```python
from build123d import *

# Parameters (mm, degrees)
SKETCH1_W           = 26
SKETCH1_H           = 18
BOSS_EXTRUDE1_DEPTH = 4
SKETCH2_W           = 3
SKETCH2_H           = 18
BOSS_EXTRUDE2_DEPTH = 35
SKETCH3_R           = 2.75
CUT_EXTRUDE1_DEPTH  = 45.519658579
FILLET1_R           = 3
FILLET2_R           = 5
SKETCH5_R           = 7
BOSS_EXTRUDE3_DEPTH = 2
CUT_EXTRUDE3_REACH  = 44.083
SKETCH7_R           = 2.25
CUT_EXTRUDE4_DEPTH  = 4
CHAMFER1_SIZE       = 2


with BuildPart() as part:
    # Sketch1 → Boss-Extrude1 (new body)
    with BuildSketch(Plane(origin=(0, 0, 0), x_dir=(0, 0, -1), z_dir=(1, 0, 0))):
        Rectangle(SKETCH1_W, SKETCH1_H)
    extrude(amount=BOSS_EXTRUDE1_DEPTH)

    # Sketch2 → Boss-Extrude2 (add)
    with BuildSketch(Plane.ZY):
        with Locations((-11.5, 0)):
            Rectangle(SKETCH2_W, SKETCH2_H)
        with Locations((11.5, 0)):
            Rectangle(SKETCH2_W, SKETCH2_H)
    extrude(amount=BOSS_EXTRUDE2_DEPTH)

    # Sketch3 → Cut-Extrude1 (cut, through all)
    with BuildSketch(Plane.XY.offset(13)):
        with Locations((-29.5, 0)):
            Circle(SKETCH3_R)
    extrude(amount=-CUT_EXTRUDE1_DEPTH, mode=Mode.SUBTRACT)

    # Fillet1
    fillet1_edges = [part.edges().sort_by_distance(p)[0] for p in [
        (4, 0, 13),
        (0, 0, -10),
        (0, 0, 10),
        (4, 0, -13),
    ]]
    fillet(fillet1_edges, radius=FILLET1_R)

    # Fillet2
    fillet2_edges = [part.edges().sort_by_distance(p)[0] for p in [
        (-35, -9, -11.5),
        (-35, 9, -11.5),
        (-35, 9, 11.5),
        (-35, -9, 11.5),
    ]]
    fillet(fillet2_edges, radius=FILLET2_R)

    # Sketch5 → Boss-Extrude3 (add)
    with BuildSketch(Plane.ZY):
        Circle(SKETCH5_R)
    extrude(amount=BOSS_EXTRUDE3_DEPTH)

    # Sketch7 → Cut-Extrude3 (cut, up to next)
    with BuildSketch(Plane(origin=(4, 0, 0), x_dir=(0, 0, -1), z_dir=(1, 0, 0)), mode=Mode.PRIVATE) as cut_extrude3_sk1:
        Circle(SKETCH7_R)
    cut_extrude3_tool1 = extrude(cut_extrude3_sk1.sketch, amount=-CUT_EXTRUDE3_REACH, mode=Mode.PRIVATE) & part.part
    add(cut_extrude3_tool1.solids().sort_by_distance((4, 0, 0))[0], mode=Mode.SUBTRACT)

    # Sketch8 → Cut-Extrude4 (cut)
    with BuildSketch(Plane.ZY.offset(2)):
        Polygon((0, 4.330127019), (-3.75, 2.165063509), (-3.75, -2.165063509), (0, -4.330127019), (3.75, -2.165063509), (3.75, 2.165063509), align=None)
    extrude(amount=-CUT_EXTRUDE4_DEPTH, mode=Mode.SUBTRACT)

    # Chamfer1
    # the kernel refuses this chamfer: 2 mm, written as the material it adds along each edge
    with BuildSketch(Plane(origin=(0, 0, 0), x_dir=(0, 0, 1), z_dir=(0, -1, 0))) as chamfer1_piece_1_section:
        Polygon((7 + CHAMFER1_SIZE, 0), (7, CHAMFER1_SIZE), (7, 0), align=None)
    chamfer1_piece_1 = revolve(axis=Axis((0, 0, 0), (-1, 0, 0)), revolution_arc=180.000000041, mode=Mode.PRIVATE)
    chamfer1_piece_1 = split(chamfer1_piece_1, bisect_by=Plane(origin=(-0.945175713, 9, -3e-09), z_dir=(0, -1, 0)), keep=Keep.TOP, mode=Mode.PRIVATE)
    chamfer1_piece_1 = split(chamfer1_piece_1, bisect_by=Plane(origin=(-2, 8.001744255, -3e-09), z_dir=(1, 0, 0)), keep=Keep.TOP, mode=Mode.PRIVATE)
    add(chamfer1_piece_1)
    with BuildSketch(Plane(origin=(0, 0, 0), x_dir=(0, -7.23525117256177e-10, -1.0), z_dir=(0, 1.0, -7.23525117256177e-10))) as chamfer1_piece_2_section:
        Polygon((7 + CHAMFER1_SIZE, 0), (7, CHAMFER1_SIZE), (7, 0), align=None)
    chamfer1_piece_2 = revolve(axis=Axis((0, 0, 0), (-1, 0, 0)), revolution_arc=179.999999959, mode=Mode.PRIVATE)
    chamfer1_piece_2 = split(chamfer1_piece_2, bisect_by=Plane(origin=(-0.945175715, -9, 3e-09), z_dir=(0, 1, 0)), keep=Keep.TOP, mode=Mode.PRIVATE)
    chamfer1_piece_2 = split(chamfer1_piece_2, bisect_by=Plane(origin=(-2, -8.001744258, 3e-09), z_dir=(1, 0, 0)), keep=Keep.TOP, mode=Mode.PRIVATE)
    add(chamfer1_piece_2)


solid = part.part
```
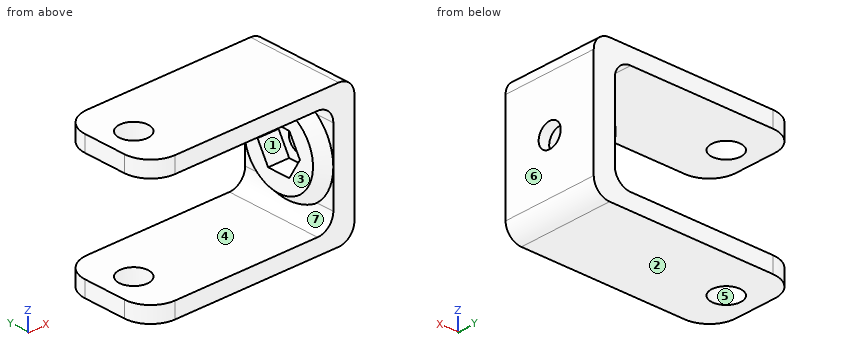
Geometry: final body of the model. Coordinates: model frame, mm. Face numbers are marked on the shaded views. A direction names the side the tool comes from. Coordinates: 2 decimals unless noted, no trailing zeros. Loops run counter-clockwise (first coordinate to the right, second up) from the corner with the lowest first, then second, coordinate; pieces in that order, holes last. Notation, with made-up numbers: (82.25, -0.5) -> (112.25, -0.5) arc R24 cw to (112.25, 17.5) -> close; hole circle Ø10 at (80.5, -11). An arc over 180 degrees is marked (long way). Use a Markdown table: item, result. Add a question column.
(1) Access query for the marked faces 1, 2 and 3. Directions: +Z, -Z, +X, -X, +Y, -Y. A direction counts if a zero-diameter tool reaches every point of the face in a straight line with its end or side. Return the directions, or none.
(2) Section query D-D, the plane y = -0.75. State how many separate pieces and enclosed holes the cut face has, plus the area to 3 significant figures.
(3) Line query: line 1 along Z through (x, y) = (-5, -7); line 2 along Y through (x, z) = (-29.5, 12.3); line 3 along Y through (x, z) = (1, -3.5). Output: solid intervals per line, ascending.
(4) Pin query (flat end, axial travel): pin 1 Ø2 at (y, z) = (-2, -1) entering from -X; pin 2 Ø8 at (y, z) = (-0.5, 1.5) entering from -X; pin 3 Ø3.5 at (y, z) = (-7.5, -5) entering from -X; pin 4 Ø3.5 at (x, y) = (-29.5, 0) entering from +Z. Return the tip coordinate at first contact, or that it passes through.
(5) Section query A-A, the plane x = -29.5. Return loops of the section in (y, z), plus the area to 3 significant figures.
(6) Mould query, pull axis X, two halves, no side actions, for the marked faces 4, 5, 6 and 7. Classes: pulls with the +X half, pulls with the -X half, needs draft (parallel to the pull), parting line crosses it, or undercut.
(7) Section query C-C, the plane z = 11.25. Return loops of the section in (x, y), plus the area to 3 significant figures.
(8) Section query B-B, the plane x = -9. Return loops of the section in (y, z), plus the area to 3 significant figures.
Answer:
| question | item | result |
|---|---|---|
| 1 | face 1 | -X |
| 1 | face 2 | -Z, +X, -X, +Y, -Y |
| 1 | face 3 | -X, +Y, -Y |
| 2 | separate pieces | 4 |
| 2 | enclosed holes | 0 |
| 2 | area | 275 mm^2 |
| 3 | line 1 | z = -13 to -10, 10 to 13 |
| 3 | line 2 | y = -9 to -2.75, 2.75 to 9 |
| 3 | line 3 | y = -9 to -2.31, 2.31 to 9 |
| 4 | pin 1 | stops at x = 2 |
| 4 | pin 2 | stops at x = -2 |
| 4 | pin 3 | stops at x = -1.74 |
| 4 | pin 4 | passes through |
| 5 | outline | (-9, -13) -> (-2.75, -13) -> (-2.75, -10) -> (-9, -10) -> close; (-9, 10) -> (-2.75, 10) -> (-2.75, 13) -> (-9, 13) -> close; (2.75, -13) -> (9, -13) -> (9, -10) -> (2.75, -10) -> close; (2.75, 10) -> (9, 10) -> (9, 13) -> (2.75, 13) -> close |
| 5 | area | 75.0 mm^2 |
| 6 | face 4 | needs draft |
| 6 | face 5 | undercut |
| 6 | face 6 | pulls with the +X half |
| 6 | face 7 | pulls with the -X half |
| 7 | outline | (-35, -4) arc R5 ccw to (-30, -9) -> (3.73, -9) -> (3.73, 9) -> (-30, 9) arc R5 ccw to (-35, 4) -> close; hole circle Ø5.5 at (-29.5, 0) |
| 7 | area | 663 mm^2 |
| 8 | outline | (-9, -13) -> (9, -13) -> (9, -10) -> (-9, -10) -> close; (-9, 10) -> (9, 10) -> (9, 13) -> (-9, 13) -> close |
| 8 | area | 108 mm^2 |
